For this review, take the finished solid that the model builds, in its own axes (mm). A direction names the side the tool comes from. Round coordinates to 2 decimals unless told otherwise and drop trailing zeros. Order: outer loops, then holes, each group sorted by start corner. A loop starts at its lowest first (then second) coordinate and runs counter-clockwise, first axis right, second up. Notation, with made-up numbers: (13, -16) -> (44, -16) arc R10 ccw to (44, 0) -> close; hole circle Ø6 at (86.5, 70). An arc over 180 degrees is marked (long way). Answer in a Markdown table with one row per item.
```python
from build123d import *

# Parameters (mm, degrees)
BOSS_EXTRU_1_DEPTH                                 = 7
ESQUISSE2_W                                        = 14
ESQUISSE2_H                                        = 5
CHAMBRAGE_POUR_VIS_T_TE_HEXAGONALE_M31_D           = 3.4
CHAMBRAGE_POUR_VIS_T_TE_HEXAGONALE_M31_DEPTH       = 12
CHAMBRAGE_POUR_VIS_T_TE_HEXAGONALE_M31_CBORE_D     = 6
CHAMBRAGE_POUR_VIS_T_TE_HEXAGONALE_M31_CBORE_DEPTH = 3.3


with BuildPart() as part:
    # Esquisse1 → Boss.-Extru.1 (new body)
    with BuildSketch(Plane(origin=(0, 0, 0), x_dir=(-1, 0, 0), z_dir=(0, 0, -1))):
        with BuildLine():
            Line((-17.5, 12.489995997), (-17.5, -12.489995997))
            ThreePointArc((-17.5, -12.489995997), (-15.202795796, -15.202795796), (-12.489995997, -17.5))
            Line((-12.489995997, -17.5), (12.489995997, -17.5))
            ThreePointArc((12.489995997, -17.5), (15.202795796, -15.202795796), (17.5, -12.489995997))
            Line((17.5, -12.489995997), (17.5, 12.489995997))
            ThreePointArc((17.5, 12.489995997), (15.202795796, 15.202795796), (12.489995997, 17.5))
            Line((12.489995997, 17.5), (-12.489995997, 17.5))
            ThreePointArc((-12.489995997, 17.5), (-15.202795796, 15.202795796), (-17.5, 12.489995997))
        make_face()
    extrude(amount=-BOSS_EXTRU_1_DEPTH)

    # Esquisse2 → Révolution1 (revolve)
    with BuildSketch(Plane(origin=(0, 0, 0), x_dir=(1, 0, 0), z_dir=(0, 1, 0))):
        with Locations((7, -9.5)):
            Rectangle(ESQUISSE2_W, ESQUISSE2_H)
    revolve(axis=Axis((0, 0, 7), (0, 0, 1)))

    # Esquisse3 → Enlèvement de matière-Révolution1 (revolve, cut)
    with BuildSketch(Plane(origin=(0, 0, 0), x_dir=(1, 0, 0), z_dir=(0, 1, 0))):
        Polygon((11, 0), (0, 0), (0, -12), (11, -12), (11, -9.5), (4, -9.5), (4, -2.5), (11, -2.5), align=None)
    revolve(axis=Axis((0, 0, 0), (0, 0, 1)), mode=Mode.SUBTRACT)

    # Chambrage pour vis à tête hexagonale M31
    with Locations(Plane(origin=(0, 0, 0), x_dir=(-1, 0, 0), z_dir=(0, 0, -1))):
        with Locations((12.374368671, 12.374368671), (-12.374368671, 12.374368671), (-12.374368671, -12.374368671), (12.374368671, -12.374368671)):
            CounterBoreHole(CHAMBRAGE_POUR_VIS_T_TE_HEXAGONALE_M31_D / 2, CHAMBRAGE_POUR_VIS_T_TE_HEXAGONALE_M31_CBORE_D / 2, CHAMBRAGE_POUR_VIS_T_TE_HEXAGONALE_M31_CBORE_DEPTH, depth=CHAMBRAGE_POUR_VIS_T_TE_HEXAGONALE_M31_DEPTH)


solid = part.part
```
Q1. Take a section at A-A, the plane x = 0. Write out the cut boundary in (y, z), then the cut area to 3 significant figures.
Answer key:
| item | result |
|---|---|
| outline | (-17.5, 0) -> (-11, 0) -> (-11, 2.5) -> (-4, 2.5) -> (-4, 9.5) -> (-11, 9.5) -> (-11, 12) -> (-14, 12) -> (-14, 7) -> (-17.5, 7) -> close; (4, 2.5) -> (11, 2.5) -> (11, 0) -> (17.5, 0) -> (17.5, 7) -> (14, 7) -> (14, 12) -> (11, 12) -> (11, 9.5) -> (4, 9.5) -> close |
| area | 219 mm^2 |
Q2. To check wall thickness, follow probe 1 along Y at (x, z) = (13.5, 5); probe 2 along X at (y, z) = (14, 3.25); probe 3 along Z at (x, y) = (-4, -2). State the ranges of each line that lie inside material, in increasing order.
Answer key:
| item | result |
|---|---|
| probe 1 | y = -16.73 to -13.65, -11.1 to 11.1, 13.65 to 16.73 |
| probe 2 | x = -16.32 to -14.9, -9.85 to 9.85, 14.9 to 16.32 |
| probe 3 | z = 2.5 to 9.5 |
Q3. Tool access review of faces 4 (the face through (0, -5, 9.5)), 5 (the face through (13.3, 13.8, 5.2)), 6 (the face through (0, -5, 2.5)): name each direction out of +Z, -Z, +X, -X, +Y, -Y from which nothing blocks a thin tool from reaching the whole face with its end or side.
Answer key:
| item | result |
|---|---|
| face 4 | +Z |
| face 5 | +Z, -Z |
| face 6 | -Z |
Q4. The part is to be moulded in two halves that separate along Y. For faces 1 (the face through (15.238, -15.168, 3.451)), 2 (the face through (-15.146, -13.523, 1.627)), 3 (the face through (12.932, -5.362, 9.465)), say which applies: +Y half, -Y half, draft (parallel to the pull), parting line (faces both ways), or undercut.
Answer key:
| item | result |
|---|---|
| face 1 | -Y half |
| face 2 | undercut |
| face 3 | parting line |
Q5. Take a section at D-D, the plane x = -13.5. Write out the cut boundary in (y, z).
Answer key:
| item | result |
|---|---|
| outline | (-16.73, 0) -> (-15.16, 0) -> (-15.16, 3.3) -> (-13.65, 3.3) -> (-13.65, 7) -> (-16.73, 7) -> close; (-11.1, 3.3) -> (-9.59, 3.3) -> (-9.59, 0) -> (9.59, 0) -> (9.59, 3.3) -> (11.1, 3.3) -> (11.1, 7) -> (3.71, 7) -> (3.71, 12) -> (-3.71, 12) -> (-3.71, 7) -> (-11.1, 7) -> close; (13.65, 3.3) -> (15.16, 3.3) -> (15.16, 0) -> (16.73, 0) -> (16.73, 7) -> (13.65, 7) -> close |
Q6. Take a section at C-C, the plane y = 13. Write out the cut boundary in (x, z).
Answer key:
| item | result |
|---|---|
| outline | (-17.12, 0) -> (-15.31, 0) -> (-15.31, 3.3) -> (-13.96, 3.3) -> (-13.96, 7) -> (-17.12, 7) -> close; (-10.79, 3.3) -> (-9.44, 3.3) -> (-9.44, 0) -> (9.44, 0) -> (9.44, 3.3) -> (10.79, 3.3) -> (10.79, 7) -> (5.2, 7) -> (5.2, 12) -> (-5.2, 12) -> (-5.2, 7) -> (-10.79, 7) -> close; (13.96, 3.3) -> (15.31, 3.3) -> (15.31, 0) -> (17.12, 0) -> (17.12, 7) -> (13.96, 7) -> close |
Q7. Clearance check with flat-ended pins moving along their axes: pin 1 Ø20 at (x, y) = (0, 0) entering from -Z; pin 2 Ø5.5 at (x, y) = (-12.37, -12.37) entering from +Z; pin 3 Ø3 at (x, y) = (12.37, 12.37) entering from -Z; pin 4 Ø3 at (y, z) = (12, 10.5) entering from -X. State where each tip first meets the part, or that it passes through.
Answer key:
| item | result |
|---|---|
| pin 1 | stops at z = 2.5 |
| pin 2 | stops at z = 7 |
| pin 3 | passes through |
| pin 4 | stops at x = -9.26 |
